Design review of the part built by this model. Coordinates are the model's own, in mm. Face numbers are marked on the shaded views. A direction names the side the tool comes from. Give positions to 0.01 mm unless a question says otherwise; leave off trailing zeros. Loops run counter-clockwise (first coordinate to the right, second up) from the corner with the lowest first, then second, coordinate; pieces in that order, holes last. Notation, with made-up numbers: (22, -33) -> (63, -33) arc R27 cw to (63, 6) -> close; hole circle Ø3 at (61, -6.5). An arc over 180 degrees is marked (long way). Answer in a Markdown table with one row per item. Add a question column.
(1) Consider section B-B on z = 266. Write out the cut boundary in (x, y).
(2) For pin 1 (0.8 mm diameter, centred on x = 0, y = -81.5, fed in from -Z); pin 2 (2 mm diameter, centred on x = -199, z = 197.5, fed in from -Y); pin 3 (2 mm diameter, centred on x = -0.5, z = 188, fed in from +Y), all flat-tipped, find the tip position at first contact; note any pin that passes through.
(3) For line 1 (Y direction, x = -19.5, z = 291), list the stretches that pass through material, from the lowest coordinate up.
(4) Consider section C-C on x = -144. Write out the cut boundary in (y, z), then the cut area to 3 significant figures.
(5) For the marked faces 1 and 2, list the 3-axis set-ups (+Z, -Z, +X, -X, +Y, -Y) from which the entire face can be reached by the end or side of a thin tool; tool diameter is ignored.
(6) Consider section A-A on y = -30. Write out the cut boundary in (x, z), then the cut area to 3 significant figures.
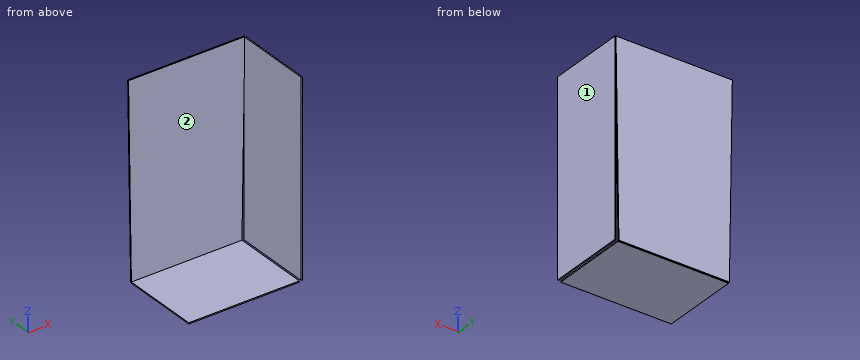
from build123d import *

# Parameters (mm, degrees)
F1_DEPTH = 1.27
F2_W     = 241.3
F2_H     = 171.45
F3_DEPTH = 1.27
F4_W     = 171.45
F4_H     = 419.1
F5_DEPTH = 1.27


with BuildPart() as f1:
    # F0 (on Front) → F1 (new body, symmetric)
    with BuildSketch(Plane.XZ):
        Polygon((-6.35, 0), (0, 419.051891), (-254, 419.051891), (-247.65, 0), align=None)
    extrude(amount=F1_DEPTH, both=True)

    # F2 (on Top) → F3 (join, symmetric)
    with BuildSketch(Plane.XY):
        with Locations((-127, -86.995)):
            Rectangle(F2_W, F2_H)
    extrude(amount=F3_DEPTH, both=True)

    # F4 (on Right) → F5 (join, symmetric)
    with BuildSketch(Plane.YZ):
        with Locations((-85.725, 209.55)):
            Rectangle(F4_W, F4_H)
    extrude(amount=F5_DEPTH, both=True)


solid = f1.part
Values follow:
| question | item | result |
|---|---|---|
| 1 | outline | (-251.68, -1.27) -> (-2.32, -1.27) -> (-2.32, 1.27) -> (-251.68, 1.27) -> close; (-1.27, -171.45) -> (1.27, -171.45) -> (1.27, 0) -> (-1.27, 0) -> close |
| 2 | pin 1 | z = 0 |
| 2 | pin 2 | y = -1.27 |
| 2 | pin 3 | y = 0 |
| 3 | line 1 | -1.27 to 1.27 |
| 4 | outline | (-172.72, -1.27) -> (-1.27, -1.27) -> (-1.27, 0) -> (1.27, 0) -> (1.27, 419.05) -> (-1.27, 419.05) -> (-1.27, 1.27) -> (-172.72, 1.27) -> close |
| 4 | area | 1,500 mm2 |
| 5 | face 1 | +Z, -Z, +X, +Y, -Y |
| 5 | face 2 | +Z, -X, -Y |
| 6 | outline | (-247.65, -1.27) -> (-6.35, -1.27) -> (-6.35, 1.27) -> (-247.65, 1.27) -> close; (-1.27, 0) -> (1.27, 0) -> (1.27, 419.1) -> (-1.27, 419.1) -> close |
| 6 | area | 1,680 mm2 |
